Model file for the job. Use its own axes, mm. A direction names the side the tool comes from. Round coordinates to 2 decimals unless told otherwise and drop trailing zeros. Order: outer loops, then holes, each group sorted by start corner. A loop starts at its lowest first (then second) coordinate and runs counter-clockwise, first axis right, second up. Notation, with made-up numbers: (85, 39) - (113, 39) arc R19 cw to (113, 49) - close; hole circle Ø7 at (-4.75, 46). An arc over 180 degrees is marked (long way). Answer as CSV lines item,"result". Start each with the question number.
1. Wall check: line 1 along X through (y, z) = (-113, 0); line 2 along Z through (x, y) = (-98, -214); line 3 along Y through (x, z) = (-61, 31.5). Give the ranges that are in metal, low to high. Write a range as [from, to].
2. 3-axis set-ups, long thin cutter, end or side, ignore diameter. For faces 1 (the face through (-20, 203, 5)), 2 (the face through (190.764, -60.075, 5.21)), 3 (the face through (7, 7, 157)): which of +Z, -Z, +X, -X, +Y, -Y reach the whole face in a straight line?
3. Band-saw the part on A-A on y = -227.5. List the corners of the cut face in (x, z), then the cut area to 3 significant figures.
4. Pull direction X, two halves, no side cores. Call faces 4 (the face through (-8, 19, 150)), 5 (the face through (-110.289, 190.367, -2.395)), 6 (the face through (193.626, 60.976, 12.605)), 7 (the face through (-235, 0, -2)): released by +X, released by -X, zero draft, split by the parting line, or undercut.
5. Pin check, flat tips, straight feed: pin 1 Ø4 at (y, z) = (151.5, 41.5) entering from -X; pin 2 Ø12 at (x, y) = (-113.75, 197.02) entering from +Z; pin 3 Ø2 at (x, y) = (100.5, 123.5) entering from -Z; pin 4 Ø24 at (x, y) = (227.5, 0) entering from +Z. Stop position of each tip, or through.
6. Band-saw the part on C-C on y = -113.75. State how many separate pieces and enclosed holes the cut face has, then the cut area to 3 significant figures.
```python
from build123d import *

# Parameters (mm, degrees)
F2_R          = 250
F2_R_2        = 200
F3_DEPTH      = 10
F3_DEPTH_BACK = 5
F4_R          = 7.5
F5_DEPTH      = 15
F7_R          = 20
F9_R          = 25.25
F10_DEPTH     = 5
F12_DEPTH     = 5


with BuildPart() as f1:
    # F0 (on Front) → F1 (revolve)
    with BuildSketch(Plane.XZ):
        with BuildLine():
            Line((200, 20), (200, 0))
            Line((200, 0), (203, 0))
            Line((203, 0), (203, 20))
            ThreePointArc((203, 20), (196.5493669363, 42.6526770285), (179.1328476019, 58.5088839444))
            ThreePointArc((179.1328476019, 58.5088839444), (92.0009441475, 89.9153591058), (0, 100.6000003082))
            Line((0, 100.6000003082), (0, 97.6))
            ThreePointArc((0, 97.6), (91.3153782925, 86.994742746), (177.7979977692, 55.8222176227))
            ThreePointArc((177.7979977692, 55.8222176227), (193.9994111035, 41.072257701), (200, 20))
        make_face()
    revolve(axis=Axis((0, 0, 99.1000001541), (0, 0, 1)))

    # F2 (on face) → F3 (join, two sides)
    with BuildSketch(Plane(origin=(0, 0, 0), x_dir=(1, 0, 0), z_dir=(0, 0, -1))) as f3_sk:
        Circle(F2_R)
        Circle(F2_R_2, mode=Mode.SUBTRACT)
    extrude(amount=F3_DEPTH)
    extrude(f3_sk.sketch, amount=-F3_DEPTH_BACK)

    # F4 (on face) → F5 (cut, through all)
    with BuildSketch(Plane.XY.offset(5)):
        with Locations((227.5, 0)):
            Circle(F4_R)
        with Locations((197.020779361, 113.75)):
            Circle(F4_R)
        with Locations((113.75, 197.020779361)):
            Circle(F4_R)
        with Locations((0, 227.5)):
            Circle(F4_R)
        with Locations((-113.75, 197.020779361)):
            Circle(F4_R)
        with Locations((-197.020779361, 113.75)):
            Circle(F4_R)
        with Locations((-227.5, 0)):
            Circle(F4_R)
        with Locations((-197.020779361, -113.75)):
            Circle(F4_R)
        with Locations((-113.75, -197.020779361)):
            Circle(F4_R)
        with Locations((0, -227.5)):
            Circle(F4_R)
        with Locations((113.75, -197.020779361)):
            Circle(F4_R)
        with Locations((197.020779361, -113.75)):
            Circle(F4_R)
    extrude(amount=-F5_DEPTH, mode=Mode.SUBTRACT)

    # F7 (on offset) → F8 (join, up to the next surface of F1)
    with BuildSketch(Plane.XY.offset(150)):
        Circle(F7_R)
    extrude(until=Until.NEXT, dir=(0, 0, -1))

    # F9 (on face) → F10 (join)
    with BuildSketch(Plane.XY.offset(150)):
        Circle(F9_R)
    extrude(amount=F10_DEPTH)

    # F11 (on face) → F12 (join)
    with BuildSketch(Plane.XY.offset(155)):
        Polygon((-14.1421356237, 14.1421356237), (0, 0), (14.1421356237, 14.1421356237), align=None)
    extrude(amount=F12_DEPTH)


solid = f1.part
```
Reply:
1,line 1,"x = [-223, -204.48], [-189.56, -165.02], [165.02, 189.56], [204.48, 223]"
1,line 2,"z = [-10, 5]"
1,line 3,"y = [-191.98, -188.7], [188.7, 191.98]"
2,face 1,"+Z"
2,face 2,"-Z"
2,face 3,"+Z, +X, -Y"
3,outline,"(-103.65, -10) - (-7.5, -10) - (-7.5, 5) - (-103.65, 5) - close; (7.5, -10) - (103.65, -10) - (103.65, 5) - (7.5, 5) - close"
3,area,"2,880 mm2"
4,face 4,"zero draft"
4,face 5,"undercut"
4,face 6,"split by the parting line"
4,face 7,"undercut"
5,pin 1,"stops at x = -129.22"
5,pin 2,"passes through"
5,pin 3,"stops at z = 64.03"
5,pin 4,"stops at z = 5"
6,separate pieces,"3"
6,enclosed holes,"0"
6,area,"2,620 mm2"
